Verification items for the finished model (mm, model axes). Face numbers are marked on the shaded views. A direction names the side the tool comes from. Coordinates: 2 decimals unless noted, no trailing zeros. Order: outer loops, then holes, each group sorted by start corner. A loop starts at its lowest first (then second) coordinate and runs counter-clockwise, first axis right, second up. Notation, with made-up numbers: (65.25, 27) - (98.25, 27) arc R30 cw to (98.25, 57) - close; hole circle Ø1 at (47, 69.25). An arc over 180 degrees is marked (long way). Answer as CSV lines item,"result". Start each with the question number.
1. Section check A-A (y = 30). Record the cut outline in (x, z).
2. Section check C-C (y = 7.5). Record the cut outline in (x, z).
3. Mould release check, pull along X, two halves, no side actions. Record for the marked faces 3, 4 and 5: pulls with the +X half, pulls with the -X half, needs draft (parallel to the pull), parting line crosses it, or undercut.
4. Section check D-D (x = 0). Record the cut outline in (y, z).
5. Set-up check for the marked faces 1 and 2: record each of +Z, -Z, +X, -X, +Y, -Y from which the full face is reachable in a straight line by a thin tool's end or side.
6. Section check B-B (z = 0). Record the cut outline in (x, y).
7. Material ranges on L1, parallel to Y at x = -6.8, z = 0; L2, parallel to Y at x = 0, z = -6.85; L3, parallel to Z at x = -4.5, y = 85.5, recorded low to high. Write a range as [from, to].
8. Go/stop test with a flat-tipped pin: pin 1 (4.5 mm diameter, centred on x = 0, y = 30, fed in from -Z). Record where the tip stops, or that it passes through.
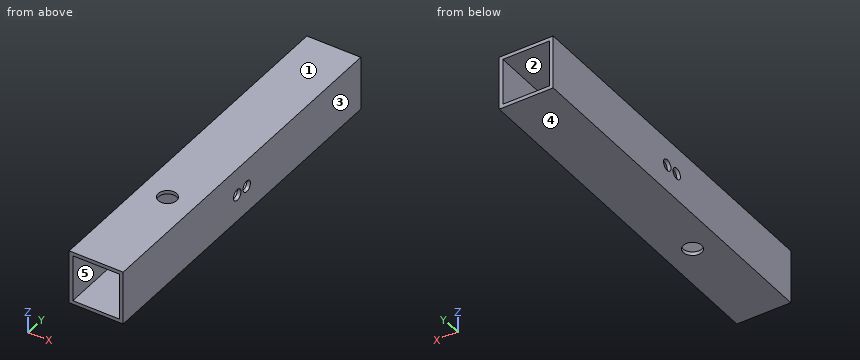
from build123d import *

# Parameters (mm, degrees)
SKETCH_1_W          = 15
SKETCH_1_H          = 15
SKETCH_1_W_2        = 13
SKETCH_1_H_2        = 13
EXTRUDE_1_DEPTH     = 100
SKETCH_2_R          = 2.55
CUT_EXTRUDE_1_DEPTH = 100
SKETCH_4_R          = 1.55
CUT_EXTRUDE_2_DEPTH = 15


with BuildPart() as part:
    # 草图1 → 凸台-拉伸1 (new body)
    with BuildSketch(Plane(origin=(0, 0, 0), x_dir=(1, 0, 0), z_dir=(0, 1, 0))):
        Rectangle(SKETCH_1_W, SKETCH_1_H)
        Rectangle(SKETCH_1_W_2, SKETCH_1_H_2, mode=Mode.SUBTRACT)
    extrude(amount=EXTRUDE_1_DEPTH)

    # 草图2 → 切除-拉伸1 (cut)
    with BuildSketch(Plane.XY.offset(7.5)):
        with Locations((0, 30)):
            Circle(SKETCH_2_R)
    extrude(amount=-CUT_EXTRUDE_1_DEPTH, mode=Mode.SUBTRACT)

    # 草图4 → 切除-拉伸2 (cut)
    with BuildSketch(Plane(origin=(7.5, 0, 0), x_dir=(0, 0, -1), z_dir=(1, 0, 0))):
        with Locations((0, 52)):
            Circle(SKETCH_4_R)
        with Locations((0, 48)):
            Circle(SKETCH_4_R)
    extrude(amount=-CUT_EXTRUDE_2_DEPTH, mode=Mode.SUBTRACT)


solid = part.part
Evaluation:
1,outline,"(-7.5, -7.5) - (-2.55, -7.5) - (-2.55, -6.5) - (-6.5, -6.5) - (-6.5, 6.5) - (-2.55, 6.5) - (-2.55, 7.5) - (-7.5, 7.5) - close; (2.55, -7.5) - (7.5, -7.5) - (7.5, 7.5) - (2.55, 7.5) - (2.55, 6.5) - (6.5, 6.5) - (6.5, -6.5) - (2.55, -6.5) - close"
2,outline,"(-7.5, -7.5) - (7.5, -7.5) - (7.5, 7.5) - (-7.5, 7.5) - close; hole (-6.5, -6.5) - (6.5, -6.5) - (6.5, 6.5) - (-6.5, 6.5) - close"
3,face 3,"pulls with the +X half"
3,face 4,"needs draft"
3,face 5,"undercut"
4,outline,"(0, -7.5) - (27.45, -7.5) - (27.45, -6.5) - (0, -6.5) - close; (0, 6.5) - (27.45, 6.5) - (27.45, 7.5) - (0, 7.5) - close; (32.55, -7.5) - (100, -7.5) - (100, -6.5) - (32.55, -6.5) - close; (32.55, 6.5) - (100, 6.5) - (100, 7.5) - (32.55, 7.5) - close"
5,face 1,"+Z, +X, -X, +Y, -Y"
5,face 2,"+Y, -Y"
6,outline,"(-7.5, 0) - (-6.5, 0) - (-6.5, 46.45) - (-7.5, 46.45) - close; (-7.5, 49.55) - (-6.5, 49.55) - (-6.5, 50.45) - (-7.5, 50.45) - close; (-7.5, 53.55) - (-6.5, 53.55) - (-6.5, 100) - (-7.5, 100) - close; (6.5, 0) - (7.5, 0) - (7.5, 46.45) - (6.5, 46.45) - close; (6.5, 49.55) - (7.5, 49.55) - (7.5, 50.45) - (6.5, 50.45) - close; (6.5, 53.55) - (7.5, 53.55) - (7.5, 100) - (6.5, 100) - close"
7,L1,"y = [0, 46.45], [49.55, 50.45], [53.55, 100]"
7,L2,"y = [0, 27.45], [32.55, 100]"
7,L3,"z = [-7.5, -6.5], [6.5, 7.5]"
8,pin 1,"passes through"
